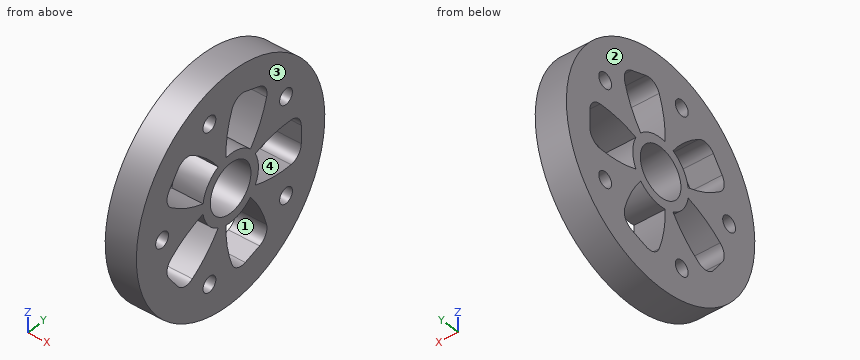
from build123d import *

# Parameters (mm, degrees)
SKETCH_1_R      = 44
SKETCH_1_R_2    = 3
SKETCH_1_R_3    = 9.5
EXTRUDE_1_DEPTH = 12


with BuildPart() as part:
    # 草图1 → 凸台-拉伸1 (new body)
    with BuildSketch(Plane(origin=(0, 0, 0), x_dir=(0, 0, -1), z_dir=(1, 0, 0))):
        Circle(SKETCH_1_R)
        with Locations((0, -32)):
            Circle(SKETCH_1_R_2, mode=Mode.SUBTRACT)
        with Locations((-30.433808521, -9.88854382)):
            Circle(SKETCH_1_R_2, mode=Mode.SUBTRACT)
        with Locations((-18.809128073, 25.88854382)):
            Circle(SKETCH_1_R_2, mode=Mode.SUBTRACT)
        with Locations((18.809128073, 25.88854382)):
            Circle(SKETCH_1_R_2, mode=Mode.SUBTRACT)
        with Locations((30.433808521, -9.88854382)):
            Circle(SKETCH_1_R_2, mode=Mode.SUBTRACT)
        Circle(SKETCH_1_R_3, mode=Mode.SUBTRACT)
        with BuildLine():
            Line((-3.5, 33), (3.5, 33))
            ThreePointArc((3.5, 33), (6.946569358, 31.62231413), (8.493822755, 28.248463863))
            ThreePointArc((8.493822755, 28.248463863), (8.076258868, 19.766783996), (6, 11.532562595))
            ThreePointArc((6, 11.532562595), (0, 13), (-6, 11.532562595))
            ThreePointArc((-6, 11.532562595), (-8.076258868, 19.766783996), (-8.493822755, 28.248463863))
            ThreePointArc((-8.493822755, 28.248463863), (-6.946569358, 31.62231413), (-3.5, 33))
        make_face(mode=Mode.SUBTRACT)
        with BuildLine():
            Line((30.303305557, 13.526258621), (32.466424518, 6.868863007))
            ThreePointArc((32.466424518, 6.868863007), (32.221215898, 3.165252414), (29.490621211, 0.651149919))
            ThreePointArc((29.490621211, 0.651149919), (21.295029967, -1.572706445), (12.822220771, -2.142581267))
            ThreePointArc((12.822220771, -2.142581267), (12.363734712, 4.017220927), (9.114016839, 9.270096928))
            ThreePointArc((9.114016839, 9.270096928), (16.303627484, 13.789250803), (24.241150054, 16.807360878))
            ThreePointArc((24.241150054, 16.807360878), (27.92799993, 16.378412522), (30.303305557, 13.526258621))
        make_face(mode=Mode.SUBTRACT)
        with BuildLine():
            Line((22.228472806, -24.640312431), (16.565353845, -28.754809197))
            ThreePointArc((16.565353845, -28.754809197), (12.967237226, -29.666080556), (9.732383503, -27.846031081))
            ThreePointArc((9.732383503, -27.846031081), (5.084793443, -20.738770033), (1.924568248, -12.856750642))
            ThreePointArc((1.924568248, -12.856750642), (7.64120828, -10.517220927), (11.632772181, -5.803327614))
            ThreePointArc((11.632772181, -5.803327614), (18.152454794, -11.24455832), (23.475677415, -17.860943579))
            ThreePointArc((23.475677415, -17.860943579), (24.207022553, -21.49989851), (22.228472806, -24.640312431))
        make_face(mode=Mode.SUBTRACT)
        with BuildLine():
            Line((-16.565353845, -28.754809197), (-22.228472806, -24.640312431))
            ThreePointArc((-22.228472806, -24.640312431), (-24.207022553, -21.49989851), (-23.475677415, -17.860943579))
            ThreePointArc((-23.475677415, -17.860943579), (-18.152454794, -11.24455832), (-11.632772181, -5.803327614))
            ThreePointArc((-11.632772181, -5.803327614), (-7.64120828, -10.517220927), (-1.924568248, -12.856750642))
            ThreePointArc((-1.924568248, -12.856750642), (-5.084793443, -20.738770033), (-9.732383503, -27.846031081))
            ThreePointArc((-9.732383503, -27.846031081), (-12.967237226, -29.666080556), (-16.565353845, -28.754809197))
        make_face(mode=Mode.SUBTRACT)
        with BuildLine():
            Line((-32.466424518, 6.868863007), (-30.303305557, 13.526258621))
            ThreePointArc((-30.303305557, 13.526258621), (-27.92799993, 16.378412522), (-24.241150054, 16.807360878))
            ThreePointArc((-24.241150054, 16.807360878), (-16.303627484, 13.789250803), (-9.114016839, 9.270096928))
            ThreePointArc((-9.114016839, 9.270096928), (-12.363734712, 4.017220927), (-12.822220771, -2.142581267))
            ThreePointArc((-12.822220771, -2.142581267), (-21.295029967, -1.572706445), (-29.490621211, 0.651149919))
            ThreePointArc((-29.490621211, 0.651149919), (-32.221215898, 3.165252414), (-32.466424518, 6.868863007))
        make_face(mode=Mode.SUBTRACT)
    extrude(amount=EXTRUDE_1_DEPTH)


solid = part.part
Can you work these out from the model? Positions are in its coordinate system, mm. Face numbers are marked on the shaded views. A direction names the side the tool comes from. Round coordinates to 2 decimals unless told otherwise and drop trailing zeros. Write each loop counter-clockwise with the first axis right and the second up, starting at its lowest first coordinate (ties: lowest second). Pieces come first, ordered by that corner, then holes. Notation, with made-up numbers: M 84,77 L 106,77 A21 ccw 106,102 Z; hole C -30,39.5 d6. An arc over 180 degrees is marked long. Use a Markdown table: item, result.
Item 1: I want a section at B-B (y = -32). List the corners of the cut face in (x, z) for me, and give its area (3 significant figures).
Found:
| item | result |
|---|---|
| outline | M 0,-30.2 L 12,-30.2 L 12,-3 L 0,-3 Z; M 0,3 L 12,3 L 12,30.2 L 0,30.2 Z |
| area | 653 mm2 |
Item 2: Which directions (+Z, -Z, +X, -X, +Y, -Y) give clear straight access to the entire face, cutting with the end or side of a thin tool? Please do the marked faces 1 and 2.
Found:
| item | result |
|---|---|
| face 1 | +X, -X |
| face 2 | +Z, -Z, -X, +Y, -Y |
Item 3: I want a section at A-A (z = 0). List the corners of the cut face in (x, y) for me.
Found:
| item | result |
|---|---|
| outline | M 0,-44 L 12,-44 L 12,-35 L 0,-35 Z; M 0,-29 L 12,-29 L 12,-9.5 L 0,-9.5 Z; M 0,9.5 L 12,9.5 L 12,13 L 0,13 Z; M 0,33 L 12,33 L 12,44 L 0,44 Z |
Item 4: We'd pull the mould along Z, two halves only. Please class the marked faces 3 and 4: released by +Z, released by -Z, zero draft, split by the parting line, or undercut.
Found:
| item | result |
|---|---|
| face 3 | zero draft |
| face 4 | undercut |
Item 5: For pin 1 Ø5.5 at (y, z) = (25.89, 18.81) entering from +X; pin 2 Ø4 at (x, z) = (8.5, -27) entering from -Y; pin 3 Ø9.5 at (y, z) = (-32, 0) entering from +X; pin 4 Ø2 at (x, z) = (7, 22.5) entering from -Y, each with a flat end and sliding along its axis, tell me the tip position at first contact or that it passes through.
Found:
| item | result |
|---|---|
| pin 1 | passes through |
| pin 2 | stops at y = -36.21 |
| pin 3 | stops at x = 12 |
| pin 4 | stops at y = -38.39 |
Item 6: If I drill on line 1 along Y through (x, z) = (6.5, 0); line 2 along Z through (x, y) = (8.5, 2); line 3 along Z through (x, y) = (8.25, -26), over which ranges is the centre line in solid material (lowest first)? Write a range as [from, to].
Found:
| item | result |
|---|---|
| line 1 | y = [-44, -35], [-29, -9.5], [9.5, 13], [33, 44] |
| line 2 | z = [-43.95, -31.45], [-12.85, -9.29], [9.29, 12.85], [31.45, 43.95] |
| line 3 | z = [-35.5, -20.36], [-8.33, 8.33], [20.36, 35.5] |
Item 7: I want a section at C-C (y = 5). List the corners of the cut face in (x, z) for me, and give its area (3 significant figures).
Found:
| item | result |
|---|---|
| outline | M 0,-43.71 L 12,-43.71 L 12,-32.7 L 0,-32.7 Z; M 0,-12 L 12,-12 L 12,-8.08 L 0,-8.08 Z; M 0,8.08 L 12,8.08 L 12,12 L 0,12 Z; M 0,32.7 L 12,32.7 L 12,43.71 L 0,43.71 Z |
| area | 358 mm2 |
Item 8: I want a section at D-D (x = 3). State how many separate pieces and enclosed holes the cut face has, and give its area (3 significant figures).
Found:
| item | result |
|---|---|
| separate pieces | 1 |
| enclosed holes | 11 |
| area | 4,060 mm2 |
